Autodesk Fusion 360 part; units mm, degrees
sketch "Esquisse1" plane through (0, 0, 0) normal (1, 0, 0) x (0, 1, 0)
  line L0 (0, 0) -> (19.5, 0)
  line L1 (19.5, 0) -> (19.5, 7.75)
  line L2 (19.5, 7.75) -> (9.5, 7.75)
  line L3 (9.5, 7.75) -> (0, 3.5)
  line L4 (0, 3.5) -> (0, 0)
  dimension "d1" = 7.75
  dimension "d2" = 19.5
  dimension "d3" = 10
  dimension "d4" = 3.5
extrude "Extrusion1" add sketch "Esquisse1" along normal blind 16.6
sketch "Esquisse2" plane through (0, 19.5, 0) normal (0, 1, 0) x (-1, 0, 0)
  line L0 (0, 0) -> (0, 7.75)
  line L1 (0, 7.75) -> (-16.6, 7.75)
  line L2 (-16.6, 7.75) -> (-16.6, 0)
  line L3 (-16.6, 0) -> (0, 0)
  line L4 (-20.05, 10.875) -> (3.45, 10.875)
  line L5 (3.45, 10.875) -> (3.45, -3.125)
  line L6 (3.45, -3.125) -> (-20.05, -3.125)
  line L7 (-20.05, -3.125) -> (-20.05, 10.875)
  dimension "d7" = 23.5
  dimension "d8" = 14
  dimension "d9" = 3.45
  dimension "d10" = 3.125
extrude "Extrusion2" add sketch "Esquisse2" along normal blind 2 contours L0 L1 L2 L3 | L4 L5 L6 L7
sketch "Esquisse3" plane through (0, 21.5, 0) normal (0, 1, 0) x (-1, 0, 0)
  line L0 (-20.05, -3.125) -> (3.45, -3.125)
  line L1 (3.45, -3.125) -> (3.45, 10.875)
  line L2 (3.45, 10.875) -> (-20.05, 10.875)
  line L3 (-20.05, 10.875) -> (-20.05, -3.125)
  line L4 (-8.3, 10.875) -> (-8.3, -3.125)
  line L5 (-14.05, 0.875) -> (-11.05, 0.875)
  line L6 (-11.05, 0.875) -> (-11.05, 3.875)
  line L7 (-11.05, 3.875) -> (-10.05, 3.875)
  line L8 (-10.05, 3.875) -> (-10.05, 5.875)
  line L9 (-10.05, 5.875) -> (-15.05, 5.875)
  line L10 (-15.05, 5.875) -> (-15.05, 3.875)
  line L11 (-15.05, 3.875) -> (-14.05, 3.875)
  line L12 (-14.05, 3.875) -> (-14.05, 0.875)
  line L13 (-1.55, 3.875) -> (-2.55, 3.875)
  line L14 (-6.55, 5.875) -> (-1.55, 5.875)
  line L15 (-6.55, 3.875) -> (-6.55, 5.875)
  line L16 (-5.55, 3.875) -> (-6.55, 3.875)
  line L17 (-5.55, 0.875) -> (-5.55, 3.875)
  line L18 (-2.55, 0.875) -> (-5.55, 0.875)
  line L19 (-2.55, 3.875) -> (-2.55, 0.875)
  line L20 (-1.55, 5.875) -> (-1.55, 3.875)
  line L21 (-14.05, 3.875) -> (-11.05, 3.875)
  line L22 (-2.55, 3.875) -> (-5.55, 3.875)
  dimension "d14" = 5
  dimension "d15" = 2
  dimension "d16" = 5
  dimension "d17" = 3
  dimension "d18" = 5
  dimension "d19" = 5
extrude "Extrusion3" cut sketch "Esquisse3" against normal blind 2 contours L5 L6 L12 L21 | L7 L8 L9 L10 L11 L21 | L13 L14 L15 L16 L20 L22 | L17 L18 L19 L22
sketch "Esquisse4" plane through (0, 21.5, 0) normal (0, 1, 0) x (-1, 0, 0)
  line L0 (-11.05, 0.875) -> (-14.05, 0.875)
  line L1 (-14.05, 0.875) -> (-14.05, 3.875)
  line L2 (-14.05, 3.875) -> (-15.05, 3.875)
  line L3 (-15.05, 3.875) -> (-15.05, 5.875)
  line L4 (-15.05, 5.875) -> (-10.05, 5.875)
  line L5 (-10.05, 5.875) -> (-10.05, 3.875)
  line L6 (-10.05, 3.875) -> (-11.05, 3.875)
  line L7 (-11.05, 3.875) -> (-11.05, 0.875)
  line L8 (-6.55, 3.875) -> (-6.55, 5.875)
  line L9 (-6.55, 5.875) -> (-1.55, 5.875)
  line L10 (-1.55, 5.875) -> (-1.55, 3.875)
  line L11 (-1.55, 3.875) -> (-2.55, 3.875)
  line L12 (-2.55, 3.875) -> (-2.55, 0.875)
  line L13 (-2.55, 0.875) -> (-5.55, 0.875)
  line L14 (-5.55, 0.875) -> (-5.55, 3.875)
  line L15 (-5.55, 3.875) -> (-6.55, 3.875)
  line L16 (-20.05, -3.125) -> (3.45, -3.125)
  line L17 (3.45, -3.125) -> (3.45, 10.875)
  line L18 (3.45, 10.875) -> (-20.05, 10.875)
  line L19 (-20.05, 10.875) -> (-20.05, -3.125)
  line L20 (-15.05, 5.875) -> (-10.05, 5.875)
  line L21 (-10.05, 5.875) -> (-10.05, 3.875)
  line L22 (-10.05, 3.875) -> (-15.05, 3.875)
  line L23 (-15.05, 3.875) -> (-15.05, 5.875)
  line L24 (-6.55, 5.875) -> (-1.55, 5.875)
  line L25 (-1.55, 5.875) -> (-1.55, 3.875)
  line L26 (-1.55, 3.875) -> (-6.55, 3.875)
  line L27 (-6.55, 3.875) -> (-6.55, 5.875)
extrude "Extrusion4" cut sketch "Esquisse4" against normal blind 5 contours L2 L3 L4 L5 L6 L20 L21 L22 L23 | L8 L9 L10 L11 L15 L24 L25 L26 L27
chamfer "Chanfrein1" [suppressed]
fillet "Congé1" [suppressed]
Design review of the part built by this model. Coordinates are the model's own, in mm. A direction names the side the tool comes from. Give positions to 0.01 mm unless a question says otherwise; leave off trailing zeros. Write each loop counter-clockwise with the first axis right and the second up, starting at its lowest first coordinate (ties: lowest second). Pieces come first, ordered by that corner, then holes. Notation, with made-up numbers: M 78,5 L 113,5 A12 cw 113,26 Z; hole C -4.75,75 d8. An arc over 180 degrees is marked long. Return JSON: item names as keys, results as strings. Group by question number.
Item 1: The part is to be moulded in two halves that separate along Z. For faces 1 (the flat face through (8, 21.5, 4)), 2 (the flat face through (14.05, 21, 2)), 3 (the flat face through (8, 15, 7.75)), say which applies: pulls with the +Z half, pulls with the -Z half, needs draft (parallel to the pull), parting line crosses it, or undercut.
Item 2: Tool access review of faces 4 (the flat face through (4, 16.5, 5)), 5 (the flat face through (8, 0, 2)): name each direction out of +Z, -Z, +X, -X, +Y, -Y from which nothing blocks a thin tool from reaching the whole face with its end or side.
Item 3: Take a section at B-B (z = 2.25). Give the boundary of the cut face in (x, y).
Item 4: Take a section at C-C (y = 12). Give the boundary of the cut face in (x, z), plus the area to 3 significant figures.
Item 5: Wall thickness on line 1 along Z through (x, y) = (1, 10.5); line 2 along Y through (x, z) = (3, -0.5); line 3 along X through (y, z) = (9, 0.75): over which ranges is each line inside the solid? List them lowest first.
Item 6: Take a section at D-D (x = 14.75). Give the boundary of the cut face in (y, z) (3 decimals), plus the area to 3 significant figures.
Item 7: Take a section at A-A (x = 12). Give the boundary of the cut face in (y, z) (3 decimals).
Item 8: Clearance check with flat-ended pins moving along their axes: pin 1 Ø4 at (x, y) = (3, 14) entering from +Z; pin 2 Ø4 at (y, z) = (11, 7.5) entering from -X; pin 3 Ø1 at (x, z) = (4.5, 4.5) entering from +Y. State where each tip first meets the part, or that it passes through.
Return value:
{
 "1": {"face 1": "needs draft", "face 2": "undercut", "face 3": "pulls with the +Z half"},
 "2": {"face 4": "+Y", "face 5": "+Z, -Z, +X, -X, -Y"},
 "3": {"outline": "M -3.45,19.5 L 0,19.5 L 0,0 L 16.6,0 L 16.6,19.5 L 20.05,19.5 L 20.05,21.5 L 14.05,21.5 L 14.05,19.5 L 11.05,19.5 L 11.05,21.5 L 5.55,21.5 L 5.55,19.5 L 2.55,19.5 L 2.55,21.5 L -3.45,21.5 Z"},
 "4": {"outline": "M 0,0 L 16.6,0 L 16.6,7.75 L 0,7.75 Z", "area": "129 mm2"},
 "5": {"line 1": "z = 0 to 7.75", "line 2": "y = 19.5 to 21.5", "line 3": "x = 0 to 16.6"},
 "6": {"outline": "M 0,0 L 19.5,0 L 19.5,-3.125 L 21.5,-3.125 L 21.5,3.875 L 16.5,3.875 L 16.5,5.875 L 21.5,5.875 L 21.5,10.875 L 19.5,10.875 L 19.5,7.75 L 9.5,7.75 L 0,3.5 Z", "area": "149 mm2"},
 "7": {"outline": "M 0,0 L 19.5,0 L 19.5,-3.125 L 21.5,-3.125 L 21.5,0.875 L 19.5,0.875 L 19.5,3.875 L 16.5,3.875 L 16.5,5.875 L 21.5,5.875 L 21.5,10.875 L 19.5,10.875 L 19.5,7.75 L 9.5,7.75 L 0,3.5 Z"},
 "8": {"pin 1": "stops at z = 7.75", "pin 2": "stops at x = 0", "pin 3": "stops at y = 16.5"}
}
